Geometry check sheet. Reference: the model listing, model coordinates, mm. A direction names the side the tool comes from. Coordinates: 2 decimals unless noted, no trailing zeros. Loops run counter-clockwise (first coordinate to the right, second up) from the corner with the lowest first, then second, coordinate; pieces in that order, holes last.
from build123d import *

# Parameters (mm, degrees)
SKETCH1_W           = 38.1
SKETCH1_H           = 38.1
BOSS_EXTRUDE1_DEPTH = 38.1
SKETCH2_R           = 5.1435
CUT_EXTRUDE1_DEPTH  = 38.1
SKETCH3_R           = 6.35
CUT_EXTRUDE2_DEPTH  = 19.05


with BuildPart() as part:
    # Sketch1 → Boss-Extrude1 (new body)
    with BuildSketch(Plane.XY):
        Rectangle(SKETCH1_W, SKETCH1_H)
    extrude(amount=BOSS_EXTRUDE1_DEPTH)

    # Sketch2 → Cut-Extrude1 (cut)
    with BuildSketch(Plane.XY.offset(38.1)):
        Circle(SKETCH2_R)
    extrude(amount=-CUT_EXTRUDE1_DEPTH, mode=Mode.SUBTRACT)

    # Sketch3 → Cut-Extrude2 (cut)
    with BuildSketch(Plane(origin=(0, 19.05, 0), x_dir=(1, 0, 0), z_dir=(0, 1, 0))):
        with Locations(Location((0, -19.05, 0), (0, 0, 270))):
            Circle(SKETCH3_R)
    extrude(amount=-CUT_EXTRUDE2_DEPTH, mode=Mode.SUBTRACT)


solid = part.part
(1) Sectioned sample at D-D on y = 1.5. Record the cut outline in (x, z).
Findings:
outline: (-19.05, 0) - (-4.92, 0) - (-4.92, 15.04) arc R6.35 cw to (-4.92, 23.06) - (-4.92, 38.1) - (-19.05, 38.1) - close; (4.92, 0) - (19.05, 0) - (19.05, 38.1) - (4.92, 38.1) - (4.92, 23.06) arc R6.35 cw to (4.92, 15.04) - close
(2) Access from +Z, -Z, +X, -X, +Y, -Y to the whole of each face (thin tool, end or side, straight path). Record for faces 5 (the flat face through (4, 5, 0)), 6 (the cylindrical face through (5.354, 9.658, 22.464)).
Findings:
face 5: -Z, +X, -X, +Y, -Y
face 6: +Y
(3) Sectioned sample at C-C on z = 12. Record the cut outline in (x, y), and give its area (3 significant figures).
Findings:
outline: (-19.05, -19.05) - (19.05, -19.05) - (19.05, 19.05) - (-19.05, 19.05) - close; hole circle Ø10.29 at (0, 0)
area: 1,370 mm2
(4) Gauge pin test, flat ends, axial feed: pin 1 Ø6 at (x, y) = (-6.5, -2.5) entering from -Z; pin 2 Ø0.6 at (x, z) = (6, 19.5) entering from +Y. Record the tip position at first contact, or that the pin passes through.
Findings:
pin 1: stops at z = 0
pin 2: stops at y = 0
(5) Sectioned sample at A-A on x = 0. Record the cut outline in (y, z), and give its area (3 significant figures).
Findings:
outline: (-19.05, 0) - (-5.14, 0) - (-5.14, 38.1) - (-19.05, 38.1) - close; (5.14, 0) - (19.05, 0) - (19.05, 12.7) - (5.14, 12.7) - close; (5.14, 25.4) - (19.05, 25.4) - (19.05, 38.1) - (5.14, 38.1) - close
area: 883 mm2
(6) Draft check along X on faces 1 (the flat face through (-19.05, 0, 19)), 2 (the flat face through (-9, 19.05, 19)), 3 (the cylindrical face through (-1.12, -5.02, 19.32)), 4 (the flat face through (19.05, 0, 19)). Enter one of: +X half, -X half, draft (parallel to the pull), parting line (faces both ways), or undercut.
Findings:
face 1: -X half
face 2: draft
face 3: undercut
face 4: +X half
(7) Sectioned sample at B-B on y = 11.5. Record the cut outline in (x, z).
Findings:
outline: (-19.05, 0) - (19.05, 0) - (19.05, 38.1) - (-19.05, 38.1) - close; hole circle Ø12.7 at (0, 19.05)
(8) Scan lines: L1, parallel to Y at x = 0, z = 10; L2, parallel to Z at x = 0, y = 11.5; L3, parallel to X at y = 11.5, z = 19.05. Record each from-to range of solid material in increasing order.
Findings:
L1: y = -19.05 to -5.14, 5.14 to 19.05
L2: z = 0 to 12.7, 25.4 to 38.1
L3: x = -19.05 to -6.35, 6.35 to 19.05
